from build123d import *


with BuildPart() as part:
    # Croquis1 → Revolución1 (revolve)
    with BuildSketch(Plane(origin=(0, 0, 0), x_dir=(0, 0, -1), z_dir=(1, 0, 0)), mode=Mode.PRIVATE) as revoluci_n1_sk:
        Polygon((25, 10), (-25, 10), (-25, 17.5), (-5, 17.5), (-5, 45), (-20, 45), (-20, 50), (-5.625229638, 50), (0, 43.29611237), (5.625229638, 50), (20, 50), (20, 45), (5, 45), (5, 17.5), (25, 17.5), align=None)
    revolve(revoluci_n1_sk.sketch.rotate(Axis((0, 0, 0), (0, 0, -1)), 90), axis=Axis((0, 0, 0), (0, 0, -1)))


solid = part.part
The model under review builds one solid part; all positions refer to its coordinate system, in mm. A direction names the side the tool comes from. Coordinates: 2 decimals unless noted, no trailing zeros. Loops run counter-clockwise (first coordinate to the right, second up) from the corner with the lowest first, then second, coordinate; pieces in that order, holes last.
(1) Tool access review of faces 4 (the cylindrical face through (20.765, 39.923, 12.605)), 5 (the conical face through (41.697, -13.131, -0.352)), 6 (the cylindrical face through (47.69, -15.02, -12.91)), 7 (the flat face through (-1, 19, -5)): name each direction out of +Z, -Z, +X, -X, +Y, -Y from which nothing blocks a thin tool from reaching the whole face with its end or side.
Determined:
face 4: +Z
face 5: none
face 6: +Z, -Z
face 7: -Z
(2) Draft analysis for pull direction Y (two halves, no side actions). For faces 1 (the conical face through (-9.46, 42.58, 0.27)), 2 (the flat face through (8, 8, -25)), 3 (the cylindrical face through (-3.794, 17.084, 14.86)), state which applies: +Y half, -Y half, draft (parallel to the pull), parting line (faces both ways), or undercut.
Determined:
face 1: parting line
face 2: draft
face 3: undercut
(3) Consider section A-A, the plane z = -9.5. Give the boundary of the cut face in (x, y).
Determined:
outline: circle Ø100 at (0, 0); circle Ø35 at (0, 0); hole circle Ø90 at (0, 0); hole circle Ø20 at (0, 0)
(4) Insertion check: P1, Ø12, axis at y = 22, z = -15, coming from the -X side; P2, Ø1, axis at x = 23.5, z = -0.5, coming from the +Y side; P3, Ø5, axis at x = 21, y = 3, coming from the -Z side. Each pin has a flat end and moves straight along its axis. Give the tip position at first contact, or say it passes through.
Determined:
P1: stops at x = -47.37
P2: stops at y = 37.84
P3: stops at z = -5
(5) Wall thickness on L1, parallel to Y at x = 0, z = 12; L2, parallel to Y at x = -2.5, z = -8.5; L3, parallel to X at y = 3.5, z = -9: over which ranges is each line inside the solid? List them lowest first.
Determined:
L1: y = -50 to -45, -17.5 to -10, 10 to 17.5, 45 to 50
L2: y = -49.94 to -44.93, -17.32 to -9.68, 9.68 to 17.32, 44.93 to 49.94
L3: x = -49.88 to -44.86, -17.15 to -9.37, 9.37 to 17.15, 44.86 to 49.88
